```python
from build123d import *

# Parameters (mm, degrees)
SKETCH_1_W            = 50
SKETCH_1_H            = 30
EXTRUDE_320_DEPTH     = 5
CUT_EXTRUDE_710_DEPTH = 31
SKETCH_8_W            = 50
SKETCH_8_H            = 30
EXTRUDE_1_DEPTH       = 2
SKETCH_11_R           = 6
CUT_EXTRUDE_2_DEPTH   = 51
SKETCH_12_R           = 1.5
CUT_EXTRUDE_3_DEPTH   = 13
SKETCH_12_3_R         = 3.2
CUT_EXTRUDE_4_DEPTH   = 5


with BuildPart() as part:
    # Эскиз1 → Extrude 320 (new body, symmetric)
    with BuildSketch(Plane.XY):
        with Locations((25, 15)):
            Rectangle(SKETCH_1_W, SKETCH_1_H)
    extrude(amount=EXTRUDE_320_DEPTH, both=True)

    # Эскиз2 → Cut-Extrude 710 (cut, through all)
    with BuildSketch(Plane(origin=(0, 30, 0), x_dir=(1, 0, 0), z_dir=(0, 1, 0))):
        Polygon((10.662267101, 0), (0, 0), (0, -5), (5.662267101, -5), align=None)
        Polygon((40, 0), (45, -5), (50, -5), (50, 0), align=None)
    extrude(amount=-CUT_EXTRUDE_710_DEPTH, mode=Mode.SUBTRACT)

    # Эскиз8 → Бобышка-Вытянуть1 (add)
    with BuildSketch(Plane(origin=(0, 0, -5), x_dir=(-1, 0, 0), z_dir=(0, 0, -1))):
        with Locations((-25, 15)):
            Rectangle(SKETCH_8_W, SKETCH_8_H)
    extrude(amount=EXTRUDE_1_DEPTH)

    # Эскиз11 → Вырез-Вытянуть2 (cut, through all)
    with BuildSketch(Plane.ZY):
        with Locations((-7, 15)):
            Circle(SKETCH_11_R)
    extrude(amount=-CUT_EXTRUDE_2_DEPTH, mode=Mode.SUBTRACT)

    # Эскиз12 → Вырез-Вытянуть3 (cut, through all)
    with BuildSketch(Plane.XY.offset(5)):
        with Locations((25.679943924, 5)):
            Circle(SKETCH_12_R)
        with Locations((25.331133551, 25)):
            Circle(SKETCH_12_R)
    extrude(amount=-CUT_EXTRUDE_3_DEPTH, mode=Mode.SUBTRACT)

    # Эскиз12<3> → Вырез-Вытянуть4 (cut)
    with BuildSketch(Plane.XY.offset(5)):
        with Locations((25.331133551, 25)):
            Circle(SKETCH_12_3_R)
        with Locations((25.679943924, 5)):
            Circle(SKETCH_12_3_R)
    extrude(amount=-CUT_EXTRUDE_4_DEPTH, mode=Mode.SUBTRACT)


solid = part.part
```
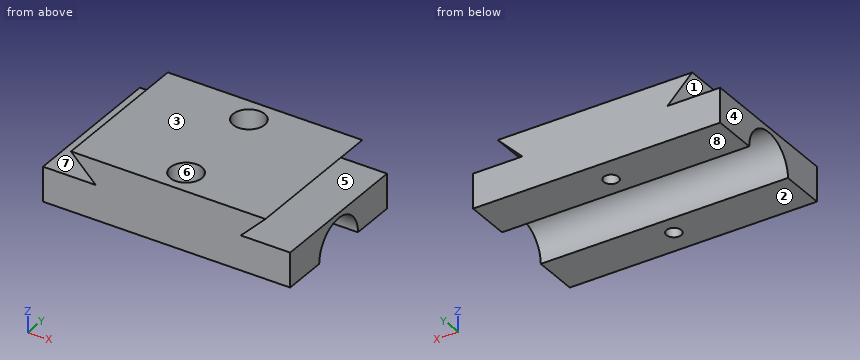
Build history of the part. All positions in model axes, mm. Face numbers are marked on the shaded views. A direction names the side the tool comes from. Coordinates: 2 decimals unless noted, no trailing zeros. Write each loop counter-clockwise with the first axis right and the second up, starting at its lowest first coordinate (ties: lowest second). Pieces come first, ordered by that corner, then holes.
1. Band-saw the part on A-A, the plane x = 43. Give the cut face in (y, z).
Answer block:
outline: (0, -7) - (9, -7) arc R6 cw to (21, -7) - (30, -7) - (30, 0) - (0, 0) - close; (0, 3) - (30, 3) - (30, 5) - (0, 5) - close
2. Band-saw the part on D-D, the plane x = 3. Give the cut face in (y, z).
Answer block:
outline: (0, -7) - (9, -7) arc R6 cw to (21, -7) - (30, -7) - (30, 0) - (0, 0) - close
3. Band-saw the part on B-B, the plane y = 5. Give the cut face in (x, z).
Answer block:
outline: (0, -7) - (24.18, -7) - (24.18, 0) - (22.48, 0) - (22.48, 5) - (5.66, 5) - (10.66, 0) - (0, 0) - close; (27.18, -7) - (50, -7) - (50, 0) - (40, 0) - (45, 5) - (28.88, 5) - (28.88, 0) - (27.18, 0) - close
4. Drop flat-ended pins along their axis: pin 1 (5 mm diameter, centred on x = 25.33, y = 25, fed in from +Z); pin 2 (7 mm diameter, centred on x = 26.5, y = 26.5, fed in from +Z); pin 3 (8 mm diameter, centred on x = 7.5, y = 16.5, fed in from -Z); pin 4 (2 mm diameter, centred on y = 21.5, z = 2, fed in from -X). Give the stop position or say it passes through.
Answer block:
pin 1: stops at z = 0
pin 2: stops at z = 5
pin 3: stops at z = -4.6
pin 4: stops at x = 7.66
5. Band-saw the part on C-C, the plane z = -5.5. Give the cut face in (x, y).
Answer block:
outline: (0, 0) - (50, 0) - (50, 9.19) - (0, 9.19) - close; (0, 20.81) - (50, 20.81) - (50, 30) - (0, 30) - close; hole circle Ø3 at (25.33, 25); hole circle Ø3 at (25.68, 5)
6. 3-axis set-ups, long thin cutter, end or side, ignore diameter. For the marked faces 5, 6, 7 and 8: which of +Z, -Z, +X, -X, +Y, -Y reach the whole face in a straight line?
Answer block:
face 5: +X, +Y, -Y
face 6: +Z
face 7: -X, +Y, -Y
face 8: -Z, +X, -X, +Y, -Y
7. Pull direction Z, two halves, no side cores. Call the marked faces 1, 2, 3 and 4: released by +Z, released by -Z, zero draft, split by the parting line, or undercut.
Answer block:
face 1: undercut
face 2: released by -Z
face 3: released by +Z
face 4: zero draft
8. Drill centre lines: probe 1 along Y at (x, z) = (24.5, -3.5); probe 2 along Z at (x, y) = (47, 6); probe 3 along Y at (x, z) = (4, -1.75). Where is each one in solid material? Low to high.
Answer block:
probe 1: y = 0 to 4.07, 5.93 to 10.13, 19.87 to 23.75, 26.25 to 30
probe 2: z = -7 to 0
probe 3: y = 0 to 12.1, 17.9 to 30
